Geometry check sheet. Reference: the model listing, model coordinates, mm. A direction names the side the tool comes from. Coordinates: 2 decimals unless noted, no trailing zeros. Loops run counter-clockwise (first coordinate to the right, second up) from the corner with the lowest first, then second, coordinate; pieces in that order, holes last. Notation, with made-up numbers: (67, 18) - (114, 18) arc R24 cw to (114, 43) - close; hole circle Ø4 at (83, -16). An arc over 180 degrees is marked (long way). Write each question's results on one line, items separated by ' | '. Start each with the question number.
(1) Sectioned sample at D-D (y = 0.5). State how many separate pieces and enclosed holes the cut face has, plus the area to 3 significant figures.
(2) Material ranges on probe 1 along Y at (x, z) = (0, 0.7) (3 decimals); probe 2 along Z at (x, y) = (5.5, -5.5); probe 3 along Y at (x, z) = (-8.25, -2), recorded low to high.
(3) Sectioned sample at B-B (x = 0). Enter the section's corners in (y, z) (3 decimals), plus the area to 3 significant figures.
(4) Go/stop test with flat-tipped pins: pin 1 Ø3.5 at (x, z) = (-6.5, 0.5) entering from -Y; pin 2 Ø3.5 at (x, z) = (6, -1) entering from -Y; pin 3 Ø1.5 at (x, y) = (-5, 0.5) entering from +Z. Record where each tip stops, or that it passes through.
(5) Access from +Z, -Z, +X, -X, +Y, -Y to the whole of each face (thin tool, end or side, straight path). Record for faces 1 (the face through (4.545, -5, 0)), 2 (the face through (-5.28, -5.34, 1.87)), 3 (the face through (0, -5, -2.5)).
(6) Sectioned sample at C-C (y = -6.25). Enter the section's corners in (x, z), plus the area to 3 significant figures.
(7) Sectioned sample at A-A (z = 0). Enter the section's corners in (x, y) (3 decimals).
from build123d import *
from OCP.BRepFilletAPI import BRepFilletAPI_MakeChamfer

# Parameters (mm, degrees)
BOSS_EXTRUDE1_DEPTH    = 2.5
BOSS_EXTRUDE2_START    = 2
BOSS_EXTRUDE2_DEPTH    = 2
CHAMFER1_SIZE          = 1
CHAMFER2_SIZE          = 1
M2_5_CLEARANCE_HOLE1_D = 2.7
CUT_EXTRUDE1_DEPTH     = 7.074630657
CHAMFER3_SIZE          = 0.4
CHAMFER3_SIZE2         = 0.292820323
CHAMFER4_SIZE          = 0.4
CHAMFER4_SIZE2         = 0.292820323
CHAMFER5_SIZE          = 1


with BuildPart() as part:
    # Sketch1 → Boss-Extrude1 (new, symmetric)
    with BuildSketch(Plane.XY):
        with BuildLine():
            Line((9.044892613, 2.649630657), (2.170272421, 2.649630657))
            ThreePointArc((2.170272421, 2.649630657), (3.095465073, 1.465851622), (3.425, 0))
            ThreePointArc((3.425, 0), (-1.465851622, -3.095465073), (-2.170272421, 2.649630657))
            Line((-2.170272421, 2.649630657), (-9.044892613, 2.649630657))
            ThreePointArc((-9.044892613, 2.649630657), (0, -9.425), (9.044892613, 2.649630657))
        make_face()
    extrude(amount=BOSS_EXTRUDE1_DEPTH, both=True)

    # Sketch2 → Boss-Extrude2 (add)
    with BuildSketch(Plane.XY.offset(2.5).offset(BOSS_EXTRUDE2_START)):
        with BuildLine():
            ThreePointArc((4.1529, 0), (3.906839776, 1.408254726), (3.197817348, 2.649630657))
            Line((3.197817348, 2.649630657), (2.170272421, 2.649630657))
            ThreePointArc((2.170272421, 2.649630657), (0, -3.425), (-2.170272421, 2.649630657))
            Line((-2.170272421, 2.649630657), (-3.197817348, 2.649630657))
            ThreePointArc((-3.197817348, 2.649630657), (-1.408254726, -3.906839776), (4.1529, 0))
        make_face()
    extrude(amount=-BOSS_EXTRUDE2_DEPTH)

    # Chamfer1
    # the kernel refuses this chamfer: 1, 0.710595202 mm, written as the material it takes off along each edge
    with BuildSketch(Plane(origin=(-2.170272421, 2.649630657, -5.071682988), x_dir=(-1, 0, 0), z_dir=(0, 0, 1))) as chamfer1_piece_1:
        with BuildLine():
            Line((CHAMFER1_SIZE, 0), (0.497857743, 0.502142257))
            ThreePointArc((0.497857743, 0.502142257), (0.261983404, 0.238250015), (0, 0))
            Line((0, 0), (CHAMFER1_SIZE, 0))
        make_face()
    extrude(amount=12.143365976, mode=Mode.SUBTRACT)

    # Chamfer2
    # the kernel refuses this chamfer: 1, 0.710595202 mm, written as the material it takes off along each edge
    with BuildSketch(Plane(origin=(2.170272421, 2.649630657, -5.071682988), x_dir=(1, 0, 0), z_dir=(0, 0, 1))) as chamfer2_piece_1:
        with BuildLine():
            Line((CHAMFER2_SIZE, 0), (0.497857743, -0.502142257))
            ThreePointArc((0.497857743, -0.502142257), (0.261983404, -0.238250015), (0, 0))
            Line((0, 0), (CHAMFER2_SIZE, 0))
        make_face()
    extrude(amount=12.143365976, mode=Mode.SUBTRACT)

    # M2.5 Clearance Hole1 (through all)
    with Locations(Plane(origin=(0, 2.649630657, 0), x_dir=(1, 0, 0), z_dir=(0, 1, 0))):
        with Locations((-7.044892613, 0), (7.044892613, 0)):
            Hole(M2_5_CLEARANCE_HOLE1_D / 2)

    # Sketch5 → Cut-Extrude1 (cut)
    with BuildSketch(Plane(origin=(0, -9.425, 0), x_dir=(-1, 0, 0), z_dir=(0, -1, 0))):
        Polygon((-12.044892613, 2.886751346), (-12.044892613, -2.886751346), (-7.044892613, -2.886751346), (-9.544892613, -1.443375673), (-9.544892613, 1.443375673), (-7.044892613, 2.886751346), align=None)
        Polygon((-4.544892613, 1.443375673), (-7.044892613, 2.886751346), (-9.544892613, 1.443375673), (-9.544892613, -1.443375673), (-7.044892613, -2.886751346), (-4.544892613, -1.443375673), align=None)
        Polygon((4.544892613, -1.443375673), (7.044892613, -2.886751346), (9.544892613, -1.443375673), (9.544892613, 1.443375673), (7.044892613, 2.886751346), (4.544892613, 1.443375673), align=None)
        Polygon((12.044892613, -2.886751346), (7.044892613, -2.886751346), (9.544892613, -1.443375673), (9.544892613, 1.443375673), (7.044892613, 2.886751346), (12.044892613, 2.886751346), align=None)
    extrude(amount=-CUT_EXTRUDE1_DEPTH, mode=Mode.SUBTRACT)

    # Chamfer3: one chamfer whose edges measure the first distance from different faces: ONE call of the kernel's chamfer builder (chamfer() names one face for all edges)
    chamfer3_edges_1 = [part.edges().sort_by_distance(p)[0] for p in [
        (6.375019632, -4.646126535, 2.5),
    ]]
    chamfer3_side_1 = [part.faces().sort_by_distance(p)[0] for p in [
        (5.422316201, -5.016137367, 1.949956418),
    ]]
    chamfer3_edges_2 = [part.edges().sort_by_distance(p)[0] for p in [
        (-6.375019632, -4.646126535, 2.5),
    ]]
    chamfer3_side_2 = [part.faces().sort_by_distance(p)[0] for p in [
        (-5.422316201, -5.016137367, 1.949956418),
    ]]
    chamfer3 = BRepFilletAPI_MakeChamfer(part.part.solid().wrapped)
    for e in chamfer3_edges_1:
        chamfer3.Add(CHAMFER3_SIZE, CHAMFER3_SIZE2, e.wrapped, chamfer3_side_1[0].wrapped)  # the first distance lies on this face
    for e in chamfer3_edges_2:
        chamfer3.Add(CHAMFER3_SIZE, CHAMFER3_SIZE2, e.wrapped, chamfer3_side_2[0].wrapped)  # the first distance lies on this face
    add(Compound.cast(chamfer3.Shape()), mode=Mode.REPLACE)

    # Chamfer4: one chamfer whose edges measure the first distance from different faces: ONE call of the kernel's chamfer builder (chamfer() names one face for all edges)
    chamfer4_edges_1 = [part.edges().sort_by_distance(p)[0] for p in [
        (6.375019632, -4.646126535, -2.5),
    ]]
    chamfer4_side_1 = [part.faces().sort_by_distance(p)[0] for p in [
        (5.422316201, -5.016137367, -1.949956418),
    ]]
    chamfer4_edges_2 = [part.edges().sort_by_distance(p)[0] for p in [
        (-6.375019632, -4.646126535, -2.5),
    ]]
    chamfer4_side_2 = [part.faces().sort_by_distance(p)[0] for p in [
        (-5.422316201, -5.016137367, -1.949956418),
    ]]
    chamfer4 = BRepFilletAPI_MakeChamfer(part.part.solid().wrapped)
    for e in chamfer4_edges_1:
        chamfer4.Add(CHAMFER4_SIZE, CHAMFER4_SIZE2, e.wrapped, chamfer4_side_1[0].wrapped)  # the first distance lies on this face
    for e in chamfer4_edges_2:
        chamfer4.Add(CHAMFER4_SIZE, CHAMFER4_SIZE2, e.wrapped, chamfer4_side_2[0].wrapped)  # the first distance lies on this face
    add(Compound.cast(chamfer4.Shape()), mode=Mode.REPLACE)

    # Chamfer5
    chamfer5_edges = [part.edges().sort_by_distance(p)[0] for p in [
        (-1.408254726, -3.906839776, 2.5),
    ]]
    chamfer(chamfer5_edges, length=CHAMFER5_SIZE)


solid = part.part
Outcome:
1) separate pieces: 2 | enclosed holes: 2 | area: 52.7 mm2
2) probe 1: y = -9.425 to -3.425 | probe 2: z = -2.5 to -1.99, 1.99 to 2.5 | probe 3: y = -2.35 to 2.65
3) outline: (-9.425, -2.5) - (-3.425, -2.5) - (-3.425, 4.5) - (-4.153, 4.5) - (-4.153, 3.5) - (-5.153, 2.5) - (-9.425, 2.5) - close | area: 32.0 mm2
4) pin 1: stops at y = -2.35 | pin 2: stops at y = -8.41 | pin 3: stops at z = 3.38
5) face 1: +X, -Y | face 2: -X, -Y | face 3: -Z, +X, -X, +Y, -Y
6) outline: (-6.08, -2.5) - (6.08, -2.5) - (6.03, -2.3) - (4.54, -1.44) - (4.54, 1.44) - (6.03, 2.3) - (6.08, 2.5) - (-6.08, 2.5) - (-6.03, 2.3) - (-4.54, 1.44) - (-4.54, -1.44) - (-6.03, -2.3) - close | area: 49.2 mm2
7) outline: (-9.127, -2.35) - (-8.395, -2.35) - (-8.395, 2.65) - (-9.045, 2.65) arc R9.425 ccw to start; (-5.695, -2.35) - (-4.545, -2.35) - (-4.545, -8.257) arc R9.425 ccw to (4.545, -8.257) - (4.545, -2.35) - (5.695, -2.35) - (5.695, 2.65) - (3.17, 2.65) - (2.668, 2.147) arc R3.425 cw (long way) to (-2.668, 2.147) - (-3.17, 2.65) - (-5.695, 2.65) - close; (8.395, -2.35) - (9.127, -2.35) arc R9.425 ccw to (9.045, 2.65) - (8.395, 2.65) - close
